```python
from build123d import *

# Parameters (mm, degrees)
CROQUIS1_W              = 249
CROQUIS1_H              = 84
SALIENTE_EXTRUIR1_DEPTH = 44.5
VACIADO1_T              = -2
CROQUIS2_W              = 20.3
CROQUIS2_H              = 20.3
CORTAR_EXTRUIR1_DEPTH   = 45
CROQUIS4_R              = 3
CORTAR_EXTRUIR2_DEPTH   = 10
CROQUIS5_W              = 249
CROQUIS5_H              = 40
CROQUIS5_H_2            = 60
SALIENTE_EXTRUIR3_DEPTH = 44.5
CROQUIS7_W              = 245
CROQUIS7_H              = 40.5
CORTAR_EXTRUIR3_DEPTH   = 180
CROQUIS8_W              = 245
CROQUIS8_H              = 180
CORTAR_EXTRUIR4_DEPTH   = 42.5
CROQUIS9_W              = 40
CROQUIS9_H              = 40
CORTAR_EXTRUIR5_DEPTH   = 2


with BuildPart() as part:
    # Croquis1 → Saliente-Extruir1 (new body)
    with BuildSketch(Plane.XY):
        with Locations((124.5, 42)):
            Rectangle(CROQUIS1_W, CROQUIS1_H)
    extrude(amount=SALIENTE_EXTRUIR1_DEPTH)

    # Vaciado1
    vaciado1_openings = [part.faces().sort_by_distance(p)[0] for p in [
        (124.5, 42, 0),
    ]]
    offset(amount=VACIADO1_T, openings=vaciado1_openings, kind=Kind.INTERSECTION)

    # Croquis2 → Cortar-Extruir1 (cut)
    with BuildSketch(Plane(origin=(0, 0, 42.5), x_dir=(-1, 0, 0), z_dir=(0, 0, -1))):
        with Locations((-100.5, 27)):
            Rectangle(CROQUIS2_W, CROQUIS2_H)
        with Locations((-33.5, 27)):
            Rectangle(CROQUIS2_W, CROQUIS2_H)
        with Locations((-215.5, 57)):
            Rectangle(CROQUIS2_W, CROQUIS2_H)
        with Locations((-148.5, 57)):
            Rectangle(CROQUIS2_W, CROQUIS2_H)
    extrude(amount=-CORTAR_EXTRUIR1_DEPTH, mode=Mode.SUBTRACT)

    # Croquis4 → Cortar-Extruir2 (cut)
    with BuildSketch(Plane.XY.offset(44.5)):
        with Locations((67, 27)):
            Circle(CROQUIS4_R)
        with Locations((182, 57)):
            Circle(CROQUIS4_R)
    extrude(amount=-CORTAR_EXTRUIR2_DEPTH, mode=Mode.SUBTRACT)

    # Croquis5 → Saliente-Extruir3 (add)
    with BuildSketch(Plane.XY.offset(44.5)):
        with Locations((124.5, 104)):
            Rectangle(CROQUIS5_W, CROQUIS5_H)
        with Locations((124.5, -30)):
            Rectangle(CROQUIS5_W, CROQUIS5_H_2)
    extrude(amount=-SALIENTE_EXTRUIR3_DEPTH)

    # Croquis7 → Cortar-Extruir3 (cut)
    with BuildSketch(Plane(origin=(0, -58, 0), x_dir=(-1, 0, 0), z_dir=(0, -1, 0))):
        with Locations((-124.5, -22.25)):
            Rectangle(CROQUIS7_W, CROQUIS7_H)
    extrude(amount=-CORTAR_EXTRUIR3_DEPTH, mode=Mode.SUBTRACT)

    # Croquis8 → Cortar-Extruir4 (cut)
    with BuildSketch(Plane(origin=(0, 0, 0), x_dir=(-1, 0, 0), z_dir=(0, 0, -1))):
        with Locations((-124.5, 32)):
            Rectangle(CROQUIS8_W, CROQUIS8_H)
    extrude(amount=-CORTAR_EXTRUIR4_DEPTH, mode=Mode.SUBTRACT)

    # Croquis9 → Cortar-Extruir5 (cut)
    with BuildSketch(Plane.XY.offset(44.5)):
        with Locations((67, -8.15)):
            Rectangle(CROQUIS9_W, CROQUIS9_H)
        with Locations((182, 21.85)):
            Rectangle(CROQUIS9_W, CROQUIS9_H)
    extrude(amount=-CORTAR_EXTRUIR5_DEPTH, mode=Mode.SUBTRACT)


solid = part.part
```
Read the model definition and answer for the solid it produces. Units are mm, in the model's axes. A direction names the side the tool comes from. Give positions to 0.01 mm unless a question says otherwise; leave off trailing zeros. Write each loop counter-clockwise with the first axis right and the second up, starting at its lowest first coordinate (ties: lowest second). Pieces come first, ordered by that corner, then holes. Notation, with made-up numbers: (8, -1) -> (55, -1) arc R19 cw to (55, 16) -> close; hole circle Ø5 at (87.25, -32). An arc over 180 degrees is marked (long way). Answer as a JSON object with one key per item and string values.
1) Section C-C on y = 57 is taken. Write down the section's boundary in (x, z), then the cut area to 3 significant figures.
Findings below:
{"outline": "(0, 0) -> (2, 0) -> (2, 42.5) -> (138.35, 42.5) -> (138.35, 44.5) -> (0, 44.5) -> close; (158.65, 42.5) -> (179, 42.5) -> (179, 44.5) -> (158.65, 44.5) -> close; (185, 42.5) -> (205.35, 42.5) -> (205.35, 44.5) -> (185, 44.5) -> close; (225.65, 42.5) -> (247, 42.5) -> (247, 0) -> (249, 0) -> (249, 44.5) -> (225.65, 44.5) -> close", "area": "575 mm^2"}
2) Section B-B on x = 67 is taken. Write down the section's boundary in (y, z), then the cut area to 3 significant figures.
Findings below:
{"outline": "(-60, 0) -> (-58, 0) -> (-58, 42.5) -> (-28.15, 42.5) -> (-28.15, 44.5) -> (-60, 44.5) -> close; (11.85, 42.5) -> (24, 42.5) -> (24, 44.5) -> (11.85, 44.5) -> close; (30, 42.5) -> (122, 42.5) -> (122, 0) -> (124, 0) -> (124, 44.5) -> (30, 44.5) -> close", "area": "446 mm^2"}
3) Straight lines are drawn through the part: probe 1 along Y at (x, z) = (182, 43); probe 2 along Y at (x, z) = (67, 43); probe 3 along X at (y, z) = (1.5, 12). For each, find the intervals that lie inside material, in ascending order. Write a range as from..to.
Findings below:
{"probe 1": "y = -60..1.85, 41.85..54, 60..124", "probe 2": "y = -60..-28.15, 11.85..24, 30..124", "probe 3": "x = 0..2, 247..249"}
4) A tool of negligible diameter and unlimited length cuts with its end or side. For faces 4 (the flat face through (2, 31, 21)), 5 (the cylindrical face through (64.6, 25.2, 43.5)), from which of +Z, -Z, +X, -X, +Y, -Y can it reach the whole face along a straight path? Write none if from no direction.
Findings below:
{"face 4": "-Z", "face 5": "+Z, -Z"}
5) Section D-D on z = 16 is taken. Write down the section's boundary in (x, y), then the cut area to 3 significant figures.
Findings below:
{"outline": "(0, -60) -> (249, -60) -> (249, 124) -> (0, 124) -> close; hole (2, -58) -> (247, -58) -> (247, 122) -> (2, 122) -> close", "area": "1,720 mm^2"}
6) For a pull along Y with two mould halves and no side action, classify faces 1 (the flat face through (0, 31, 23)), 2 (the flat face through (123, -60, 23)), 3 (the flat face through (247, 31, 21)) as pulls with the +Y half, pulls with the -Y half, needs draft (parallel to the pull), parting line crosses it, or undercut.
Findings below:
{"face 1": "needs draft", "face 2": "pulls with the -Y half", "face 3": "undercut"}
7) Section A-A on y = 27 is taken. Write down the section's boundary in (x, z), then the cut area to 3 significant figures.
Findings below:
{"outline": "(0, 0) -> (2, 0) -> (2, 42.5) -> (23.35, 42.5) -> (23.35, 44.5) -> (0, 44.5) -> close; (43.65, 42.5) -> (64, 42.5) -> (64, 44.5) -> (43.65, 44.5) -> close; (70, 42.5) -> (90.35, 42.5) -> (90.35, 44.5) -> (70, 44.5) -> close; (110.65, 42.5) -> (162, 42.5) -> (162, 44.5) -> (110.65, 44.5) -> close; (202, 42.5) -> (247, 42.5) -> (247, 0) -> (249, 0) -> (249, 44.5) -> (202, 44.5) -> close", "area": "495 mm^2"}
8) A flat-ended cylindrical pin translates along its axis: pin 1 Ø10 at (x, y) = (109.5, -16) entering from -Z. Find the tip coordinate at first contact, or state that the pin passes through.
Findings below:
{"pin 1": "stops at z = 42.5"}
